Input: part model. Units: mm. Frame: model coordinates. Round coordinates to 2 decimals unless told otherwise and drop trailing zeros. Loops run counter-clockwise (first coordinate to the right, second up) from the corner with the lowest first, then second, coordinate; pieces in that order, holes last.
(1) First-contact query: pin 1 Ø1.5 at (y, z) = (6, -7.5) entering from -X; pin 2 Ø4 at (x, y) = (-1.5, 4.5) entering from +Z; pin 3 Ø5 at (y, z) = (1.5, -12.5) entering from -X; pin 4 Ø10 at (x, z) = (-10, -4) entering from -Y. Flat tips, straight axial feed; report the tip coordinate or a pass-through.
(2) Line query: line 1 (Y direction, x = 43, z = -2); line 2 (X direction, y = -0.75, z = -12.25); line 3 (X direction, y = 2.5, z = 5.5). Output: solid intervals per line, ascending.
(3) Cut plane B-B, the plane x = 25. Output: boundary loops of the cut face in (y, z).
(4) Cut plane C-C, the plane z = 10.75. Output: boundary loops of the cut face in (x, y) (3 decimals), and give its area (3 significant figures).
(5) Cut plane D-D, the plane y = 10.25. Output: boundary loops of the cut face in (x, z), and give its area (3 significant figures).
(6) Cut plane A-A, the plane y = -2.25. Output: boundary loops of the cut face in (x, z), and give its area (3 significant figures).
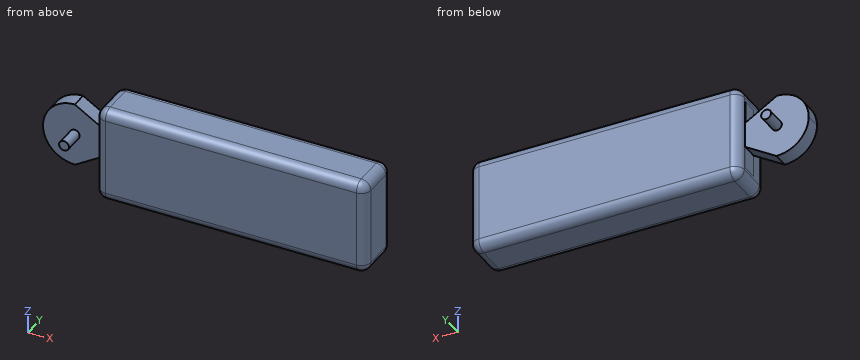
from build123d import *

# Parameters (mm, degrees)
SKETCH1_W                = 20
SKETCH1_H                = 22
BOSS_EXTRUDE1_DEPTH      = 5
BOSS_EXTRUDE2_DEPTH      = 6.5
BOSS_EXTRUDE2_DEPTH_BACK = 11.5
SKETCH2_R                = 1.55
SKETCH8_W                = 30
SKETCH8_H                = 15
BOSS_EXTRUDE3_DEPTH      = 85
FILLET1_R                = 3
FILLET2_R                = 3
FILLET3_R                = 3
FILLET4_R                = 3
FILLET5_R                = 3
FILLET6_R                = 3
CUT_EXTRUDE1_DEPTH       = 20
CUT_EXTRUDE2_DEPTH       = 20


with BuildPart() as part:
    # Sketch1 → Boss-Extrude1 (new body)
    with BuildSketch(Plane(origin=(8.035400608, 0, 0), x_dir=(1, 0, 0), z_dir=(0, 1, 0))):
        with Locations((-13.726235741, 2.992395437)):
            Rectangle(SKETCH1_W, SKETCH1_H)
    extrude(amount=BOSS_EXTRUDE1_DEPTH)

    # Sketch2 → Boss-Extrude2 (add, two sides: drawn at the far end of the back side and taken through both)
    with BuildSketch(Plane(origin=(8.035400608, 5, 0), x_dir=(1, 0, 0), z_dir=(0, 1, 0)).offset(-BOSS_EXTRUDE2_DEPTH_BACK)):
        with Locations(Location((-13.726235741, 2.992395437, 0), (0, 0, 270))):
            Circle(SKETCH2_R)
    extrude(amount=BOSS_EXTRUDE2_DEPTH + BOSS_EXTRUDE2_DEPTH_BACK)

    # Sketch8 → Boss-Extrude3 (add)
    with BuildSketch(Plane(origin=(4.309164866, 0, 0), x_dir=(0, 0, -1), z_dir=(1, 0, 0))):
        with Locations((2.837033874, 1)):
            Rectangle(SKETCH8_W, SKETCH8_H)
    extrude(amount=BOSS_EXTRUDE3_DEPTH)

    # Fillet1
    fillet1_edges = [part.edges().sort_by_distance(p)[0] for p in [
        (46.809164866, -6.5, 12.162966126),
    ]]
    fillet(fillet1_edges, radius=FILLET1_R)

    # Fillet2
    fillet2_edges = [part.edges().sort_by_distance(p)[0] for p in [
        (46.809164866, 8.5, 12.162966126),
    ]]
    fillet(fillet2_edges, radius=FILLET2_R)

    # Fillet3
    fillet3_edges = [part.edges().sort_by_distance(p)[0] for p in [
        (46.809164866, 8.5, -17.837033874),
    ]]
    fillet(fillet3_edges, radius=FILLET3_R)

    # Fillet4
    fillet4_edges = [part.edges().sort_by_distance(p)[0] for p in [
        (46.809164866, -6.5, -17.837033874),
    ]]
    fillet(fillet4_edges, radius=FILLET4_R)

    # Fillet5
    fillet5_edges = [part.edges().sort_by_distance(p)[0] for p in [
        (89.309164866, -6.5, -2.837033874),
        (89.309164866, -5.621320344, 11.284286469),
        (89.309164866, 1, 12.162966126),
        (89.309164866, 7.621320344, 11.284286469),
        (89.309164866, 8.5, -2.837033874),
        (89.309164866, 7.621320344, -16.958354218),
        (89.309164866, 1, -17.837033874),
        (89.309164866, -5.621320344, -16.958354218),
    ]]
    fillet(fillet5_edges, radius=FILLET5_R)

    # Fillet6
    fillet6_edges = [part.edges().sort_by_distance(p)[0] for p in [
        (4.309164866, -6.5, -2.837033874),
        (4.309164866, -5.621320344, 11.284286469),
        (4.309164866, 1, 12.162966126),
        (4.309164866, 7.621320344, 11.284286469),
        (4.309164866, 8.5, -2.837033874),
        (4.309164866, 7.621320344, -16.958354218),
        (4.309164866, 1, -17.837033874),
        (4.309164866, -5.621320344, -16.958354218),
    ]]
    fillet(fillet6_edges, radius=FILLET6_R)

    # Sketch7 → Cut-Extrude1 (cut)
    with BuildSketch(Plane(origin=(8.035400608, 11.5, 0), x_dir=(1, 0, 0), z_dir=(0, 1, 0))):
        with BuildLine():
            ThreePointArc((-13.726235741, -7.007604563), (-20.797303553, -4.078672375), (-23.726235741, 2.992395437))
            Line((-23.726235741, 2.992395437), (-23.726235741, -8.007604563))
            Line((-23.726235741, -8.007604563), (-3.820368823, -8.007604563))
            Line((-3.820368823, -8.007604563), (-3.820368823, -1.007604563))
            Line((-3.820368823, -1.007604563), (-13.726235741, -7.007604563))
        make_face()
    extrude(amount=-CUT_EXTRUDE1_DEPTH, mode=Mode.SUBTRACT)

    # Sketch7_4 → Cut-Extrude2 (cut)
    with BuildSketch(Plane(origin=(8.035400608, 11.5, 0), x_dir=(1, 0, 0), z_dir=(0, 1, 0))):
        Polygon((-4.043777376, 13.992395437), (-13.535691963, 13.992395437), (-13.535691963, 12.990579926), (-3.756109018, 7.010662038), (-3.726235741, 13.992395437), align=None)
        with BuildLine():
            Line((-13.535691963, 13.992395437), (-23.726235741, 13.992395437))
            Line((-23.726235741, 13.992395437), (-23.726235741, 2.992395437))
            ThreePointArc((-23.726235741, 2.992395437), (-20.729612149, 10.130512759), (-13.535691963, 12.990579926))
            Line((-13.535691963, 12.990579926), (-13.535691963, 13.992395437))
        make_face()
    extrude(amount=-CUT_EXTRUDE2_DEPTH, mode=Mode.SUBTRACT)


solid = part.part
Reported:
1. pin 1: stops at x = 4.31
1. pin 2: stops at z = 5.68
1. pin 3: stops at x = -12.82
1. pin 4: stops at y = -6.5
2. line 1: y = -6.5 to 8.5
2. line 2: x = 4.31 to 89.31
2. line 3: x = -10.97 to -3.2, 4.22 to 89.31
3. outline: (-6.5, -14.84) arc R3 ccw to (-3.5, -17.84) - (5.5, -17.84) arc R3 ccw to (8.5, -14.84) - (8.5, 9.16) arc R3 ccw to (5.5, 12.16) - (-3.5, 12.16) arc R3 ccw to (-6.5, 9.16) - close
4. outline: (4.763, -3.5) arc R2.546 ccw to (7.309, -6.046) - (86.309, -6.046) arc R2.546 ccw to (88.855, -3.5) - (88.855, 5.5) arc R2.546 ccw to (86.309, 8.046) - (7.309, 8.046) arc R2.546 ccw to (4.763, 5.5) - close
4. area: 1,180 mm2
5. outline: circle Ø3.1 at (-5.69, -2.99)
5. area: 7.55 mm2
6. outline: circle Ø3.1 at (-5.69, -2.99); (4.31, -14.84) arc R3 ccw to (7.31, -17.84) - (86.31, -17.84) arc R3 ccw to (89.31, -14.84) - (89.31, 9.16) arc R3 ccw to (86.31, 12.16) - (7.31, 12.16) arc R3 ccw to (4.31, 9.16) - close
6. area: 2,550 mm2
